For this review, take the finished solid that the model builds, in its own axes (mm). Face numbers are marked on the shaded views. Give positions to 0.01 mm unless a question says otherwise; leave off trailing zeros. Loops run counter-clockwise (first coordinate to the right, second up) from the corner with the lowest first, then second, coordinate; pieces in that order, holes last. Notation, with made-up numbers: (89, 78) - (121, 78) arc R29 cw to (121, 102) - close; hole circle Ø9 at (-13, 9.5). An arc over 180 degrees is marked (long way). Put each result on its own line as item: value.
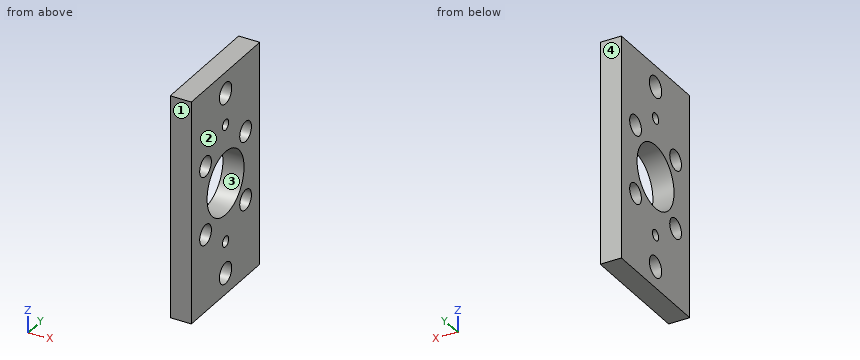
Autodesk Inventor part; units mm, degrees
ref_plane "YZ Plane" through (0, 0, 0) normal (1, 0, 0) x (0, 1, 0)
ref_plane "XZ Plane" through (0, 0, 0) normal (0, 1, 0) x (-1, 0, 0)
ref_plane "XY Plane" through (0, 0, 0) normal (0, 0, 1) x (1, 0, 0)
sketch "Sketch1" plane through (0, 0, 0) normal (1, 0, 0) x (0, 1, 0)
  line L0 (-6, -12.5) -> (-6, -12.9)
  arc A0 (-6, -12.9) -> (-5.6, -13.3) centre (-5.6, -12.9) ccw
  line L1 (-5.6, -13.3) -> (-4.9, -13.3)
  arc A1 (-4.9, -13.3) -> (-4.7, -13.1) centre (-4.9, -13.1) ccw
  line L2 (-4.7, -13.1) -> (-4.7, -12.85)
  arc A2 (-4.5, -12.65) -> (-4.7, -12.85) centre (-4.5, -12.85) ccw
  line L3 (-4.5, -12.65) -> (-1.8, -12.65)
  arc A3 (-1.4, -13.05) -> (-1.8, -12.65) centre (-1.8, -13.05) ccw
  line L4 (-1.4, -13.05) -> (-1.4, -18.75)
  line L5 (-1.8, -19.15) -> (-4.5, -19.15)
  arc A4 (-1.8, -19.15) -> (-1.4, -18.75) centre (-1.8, -18.75) ccw
  arc A5 (-4.7, -18.95) -> (-4.5, -19.15) centre (-4.5, -18.95) ccw
  line L6 (-4.7, -18.95) -> (-4.7, -18.7)
  arc A6 (-4.7, -18.7) -> (-4.9, -18.5) centre (-4.9, -18.7) ccw
  line L7 (-4.9, -18.5) -> (-5.6, -18.5)
  arc A7 (-5.6, -18.5) -> (-6, -18.9) centre (-5.6, -18.9) ccw
  line L8 (-6, -18.9) -> (-6, -19.5)
  line L9 (-6.5, -6.5) -> (-6.5, -12.5)
  line L10 (-6.5, -12.5) -> (-2.5, -12.5)
  line L11 (-1.05, -19.5) -> (-6.5, -19.5)
  line L12 (-6.5, -19.5) -> (-6.5, -26)
  line L13 (-6.5, -26) -> (-1.05, -26)
  line L14 (-6, -26) -> (-6, -26.6)
  arc A8 (-6, -26.6) -> (-5.6, -27) centre (-5.6, -26.6) ccw
  line L15 (-5.6, -27) -> (-4.9, -27)
  arc A9 (-4.9, -27) -> (-4.7, -26.8) centre (-4.9, -26.8) ccw
  arc A10 (-4.5, -26.35) -> (-4.7, -26.55) centre (-4.5, -26.55) ccw
  line L16 (-4.7, -26.8) -> (-4.7, -26.55)
  line L17 (-4.5, -26.35) -> (-1.8, -26.35)
  arc A11 (-1.4, -26.75) -> (-1.8, -26.35) centre (-1.8, -26.75) ccw
  line L18 (-1.4, -26.75) -> (-1.4, -32.45)
  arc A12 (-1.8, -32.85) -> (-1.4, -32.45) centre (-1.8, -32.45) ccw
  line L19 (-1.8, -32.85) -> (-4.5, -32.85)
  arc A13 (-4.7, -32.65) -> (-4.5, -32.85) centre (-4.5, -32.65) ccw
  line L20 (-4.7, -32.65) -> (-4.7, -32.4)
  arc A14 (-4.7, -32.4) -> (-4.9, -32.2) centre (-4.9, -32.4) ccw
  line L21 (-4.9, -32.2) -> (-5.6, -32.2)
  arc A15 (-5.6, -32.2) -> (-6, -32.6) centre (-5.6, -32.6) ccw
  line L22 (-6, -32.6) -> (-6, -33)
  line L23 (-2.5, -33) -> (-6.5, -33)
  line L24 (-6.5, -33) -> (-6.5, -39)
  line L25 (32.5, 0) -> (0, 0)
  circle A16 centre (0, -6.5) radius 4.75
  circle A17 centre (32.5, -6.5) radius 4.75
  circle A18 centre (0, -39) radius 4.75
  circle A19 centre (32.5, -39) radius 4.75
  line L26 (39, -26) -> (39, -19.5)
  line L27 (39, -12.5) -> (39, -6.5)
  line L28 (39, -39) -> (39, -33)
  line L29 (26.5, -45.5) -> (32.5, -45.5)
  line L30 (0, -45.5) -> (6, -45.5)
  line L31 (13, -45.5) -> (19.5, -45.5)
  circle A20 centre (16.2588, 5.0016) radius 2.5
  circle A21 centre (16.25, -50.5) radius 2.5
  line L32 (44, 10) -> (-11.5, 10)
  line L33 (-11.5, 10) -> (-11.5, -55.5)
  line L34 (-11.5, -55.5) -> (44, -55.5)
  line L35 (44, -55.5) -> (44, 10)
  line L36 (44, 10) -> (-11.5, 10)
  line L37 (-11.5, 10) -> (-11.5, 30)
  line L38 (-11.5, 30) -> (44, 30)
  line L39 (44, 30) -> (44, 10)
  line L40 (44, -55.5) -> (-11.5, -55.5)
  line L41 (-11.5, -55.5) -> (-11.5, -75.5)
  line L42 (-11.5, -75.5) -> (44, -75.5)
  line L43 (44, -75.5) -> (44, -55.5)
  circle A22 centre (16.25, 20) radius 5
  circle A23 centre (16.25, -65.5) radius 5
  circle A24 centre (16.25, -22.75) radius 15
  circle A25 centre (16.25, -22.75) radius 5
  point P0 (24.75, -17.8425)
  point P1 (-11.5, 10)
  dimension "d0" = 20
  dimension "d1" = 20
  dimension "d2" = 10
  dimension "d3" = 10
extrude "Extrusion2" add sketch "Sketch1" along normal blind 10 contours L35 L34 L33 L32 | L32 L37 L38 L39 | L43 L42 L41 L34
properties part number "PlacaSuperiorHidráulicos_CPY"
1) Wall thickness on line 1 (Y direction, x = 1, z = -35.5); line 2 (Z direction, x = 9, y = 15); line 3 (Z direction, x = 4.75, y = 18.5): over which ranges is each line inside the solid? List them lowest first.
Geometry check:
line 1: y = -11.5 to -3.21, 3.21 to 8.35, 24.15 to 29.29, 35.71 to 44
line 2: z = -75.5 to -70.34, -60.66 to -52.67, -48.33 to -37.7, -7.8 to 2.84, 7.16 to 15.16, 24.84 to 30
line 3: z = -75.5 to -69.97, -61.03 to -51.59, -49.41 to -37.58, -7.92 to 3.89, 6.11 to 15.53, 24.47 to 30
2) Take a section at A-A on z = -39. State the section outline as (x, y) points.
Geometry check:
outline: (0, -11.5) - (10, -11.5) - (10, -4.75) - (0, -4.75) - close; (0, 4.75) - (10, 4.75) - (10, 27.75) - (0, 27.75) - close; (0, 37.25) - (10, 37.25) - (10, 44) - (0, 44) - close
3) Take a section at D-D on x = 3.75. State how many separate pieces and enclosed holes the cut face has, and give its area (3 significant figures).
Geometry check:
separate pieces: 1
enclosed holes: 9
area: 4,670 mm²
4) Draft analysis for pull direction Y (two halves, no side actions). For the marked faces 1, 2, 3 and 4, state which applies: pulls with the +Y half, pulls with the -Y half, needs draft (parallel to the pull), parting line crosses it, or undercut.
Geometry check:
face 1: pulls with the -Y half
face 2: needs draft
face 3: undercut
face 4: pulls with the +Y half
5) Take a section at B-B on y = 32.5. State the section outline as (x, z) points.
Geometry check:
outline: (0, -75.5) - (10, -75.5) - (10, -43.75) - (0, -43.75) - close; (0, -34.25) - (10, -34.25) - (10, -11.25) - (0, -11.25) - close; (0, -1.75) - (10, -1.75) - (10, 30) - (0, 30) - close
6) Take a section at C-C on z = 23. State the section outline as (x, y) points, and give its area (3 significant figures).
Geometry check:
outline: (0, -11.5) - (10, -11.5) - (10, 12.25) - (0, 12.25) - close; (0, 20.25) - (10, 20.25) - (10, 44) - (0, 44) - close
area: 475 mm²
